```python
from build123d import *

# Parameters (mm, degrees)
F1_DEPTH = 40.64
F3_DEPTH = 38.608
F5_DEPTH = 4.7752
F6_R     = 1.35255
F7_DEPTH = 4.7752


# Not quite as in the source:
# - a feature names something its author has since deleted; it is built from what else it names


with BuildPart() as f1:
    # F0 (on Top) → F1 (new body)
    with BuildSketch(Plane.XY):
        with BuildLine():
            ThreePointArc((0, 2), (0.5857864376, 0.5857864376), (2, 0))
            Line((2, 0), (50.07, 0))
            ThreePointArc((50.07, 0), (51.4842135624, 0.5857864376), (52.07, 2))
            Line((52.07, 2), (52.07, 36.1))
            ThreePointArc((52.07, 36.1), (51.4842135624, 37.5142135624), (50.07, 38.1))
            Line((50.07, 38.1), (2, 38.1))
            ThreePointArc((2, 38.1), (0.5857864376, 37.5142135624), (0, 36.1))
            Line((0, 36.1), (0, 2))
        make_face()
    extrude(amount=F1_DEPTH)

    # F2 (on face) → F3 (cut)
    with BuildSketch(Plane.XY.offset(40.64)):
        with BuildLine():
            Line((49.27, 36.3), (2.8, 36.3))
            ThreePointArc((2.8, 36.3), (2.0928932188, 36.0071067812), (1.8, 35.3))
            Line((1.8, 35.3), (1.8, 2.8))
            ThreePointArc((1.8, 2.8), (2.0928932188, 2.0928932188), (2.8, 1.8))
            Line((2.8, 1.8), (49.27, 1.8))
            ThreePointArc((49.27, 1.8), (49.9771067812, 2.0928932188), (50.27, 2.8))
            Line((50.27, 2.8), (50.27, 35.3))
            ThreePointArc((50.27, 35.3), (49.9771067812, 36.0071067812), (49.27, 36.3))
        make_face()
    extrude(amount=-F3_DEPTH, mode=Mode.SUBTRACT)

    # F4 (on face) → F5 (join)
    with BuildSketch(Plane(origin=(0, 0, 0), x_dir=(1, 0, 0), z_dir=(0, 0, -1))):
        with BuildLine():
            ThreePointArc((52.07, -2), (51.4842135624, -0.5857864376), (50.07, 0))
            Line((50.07, 0), (46.26, 0))
            Line((46.26, 0), (46.26, -2))
            ThreePointArc((46.26, -2), (47.3759231637, -4.6940768363), (50.07, -5.81))
            Line((50.07, -5.81), (52.07, -5.81))
            Line((52.07, -5.81), (52.07, -2))
        make_face()
        with BuildLine():
            Line((46.26, -36.1), (46.26, -38.1))
            Line((46.26, -38.1), (50.07, -38.1))
            ThreePointArc((50.07, -38.1), (51.4842135624, -37.5142135624), (52.07, -36.1))
            Line((52.07, -36.1), (52.07, -32.29))
            Line((52.07, -32.29), (50.07, -32.29))
            ThreePointArc((50.07, -32.29), (47.3759231637, -33.4059231637), (46.26, -36.1))
        make_face()
        with BuildLine():
            ThreePointArc((5.81, -36.1), (4.6940768363, -33.4059231637), (2, -32.29))
            Line((2, -32.29), (0, -32.29))
            Line((0, -32.29), (0, -36.1))
            ThreePointArc((0, -36.1), (0.5857864376, -37.5142135624), (2, -38.1))
            Line((2, -38.1), (5.81, -38.1))
            Line((5.81, -38.1), (5.81, -36.1))
        make_face()
        with BuildLine():
            Line((5.81, 0), (2, 0))
            ThreePointArc((2, 0), (0.5857864376, -0.5857864376), (0, -2))
            Line((0, -2), (0, -5.81))
            Line((0, -5.81), (2, -5.81))
            ThreePointArc((2, -5.81), (4.6940768363, -4.6940768363), (5.81, -2))
            Line((5.81, -2), (5.81, 0))
        make_face()
    extrude(amount=-F5_DEPTH)

    # F6 (on face) → F7 (cut, through all)
    with BuildSketch(Plane(origin=(0, 0, 0), x_dir=(1, 0, 0), z_dir=(0, 0, -1))):
        with Locations((48.7198709242, -3.3501290758)):
            Circle(F6_R)
        with Locations((3.3501290758, -3.3501290758)):
            Circle(F6_R)
        with Locations((3.3501290758, -34.7498709242)):
            Circle(F6_R)
        with Locations((48.7198709242, -34.7498709242)):
            Circle(F6_R)
    extrude(amount=-F7_DEPTH, mode=Mode.SUBTRACT)


solid = f1.part
```
Design review of the part built by this model. Coordinates are the model's own, in mm. A direction names the side the tool comes from. Coordinates: 2 decimals unless noted, no trailing zeros. Order: outer loops, then holes, each group sorted by start corner. A loop starts at its lowest first (then second) coordinate and runs counter-clockwise, first axis right, second up.
1) Wall thickness on line 1 along X through (y, z) = (20.5, 27.5); line 2 along Y through (x, z) = (43, 29); line 3 along Z through (x, y) = (45.5, 7): over which ranges is each line inside the solid? List them lowest first.
2) Clearance check with flat-ended pins moving along their axes: pin 1 (3 mm diameter, centred on x = 47.5, y = 34, fed in from +Z); pin 2 (10 mm diameter, centred on x = 11.5, y = 12.5, fed in from +Z). State where each tip first meets the part, or that it passes through.
3) Take a section at C-C, the plane x = 19. Give the boundary of the cut face in (y, z).
4) Take a section at D-D, the plane z = 3.5. Give the boundary of the cut face in (x, y).
5) Take a section at B-B, the plane y = 11.5. Give the boundary of the cut face in (x, z), and give its area (3 significant figures).
6) Mouldability with a two-part tool opening along X and no side actions: class faces 1 (the cylindrical face through (4.64, 2.94, 2.35)), 2 (the flat face through (52.07, 19, 20)), 3 (the flat face through (26, 0, 20)) as +X half, -X half, draft (parallel to the pull), parting line (faces both ways), or undercut.
7) Take a section at A-A, the plane z = 24.5. Give the boundary of the cut face in (x, y), and give its area (3 significant figures).
8) For faces 4 (the cylindrical face through (51.5, 0.6, 20)), 5 (the flat face through (47, 35, 4.775)), list the 3-axis set-ups (+Z, -Z, +X, -X, +Y, -Y) from which the entire face can be reached by the end or side of a thin tool; tool diameter is ignored.
Returned:
1. line 1: x = 0 to 1.8, 50.27 to 52.07
1. line 2: y = 0 to 1.8, 36.3 to 38.1
1. line 3: z = 0 to 2.03
2. pin 1: stops at z = 4.78
2. pin 2: stops at z = 2.03
3. outline: (0, 0) - (38.1, 0) - (38.1, 40.64) - (36.3, 40.64) - (36.3, 2.03) - (1.8, 2.03) - (1.8, 40.64) - (0, 40.64) - close
4. outline: (0, 2) arc R2 ccw to (2, 0) - (50.07, 0) arc R2 ccw to (52.07, 2) - (52.07, 36.1) arc R2 ccw to (50.07, 38.1) - (2, 38.1) arc R2 ccw to (0, 36.1) - close; hole (1.8, 5.81) - (2, 5.81) arc R3.81 cw to (5.81, 2) - (5.81, 1.8) - (46.26, 1.8) - (46.26, 2) arc R3.81 cw to (50.07, 5.81) - (50.27, 5.81) - (50.27, 32.29) - (50.07, 32.29) arc R3.81 cw to (46.26, 36.1) - (46.26, 36.3) - (5.81, 36.3) - (5.81, 36.1) arc R3.81 cw to (2, 32.29) - (1.8, 32.29) - close; hole circle Ø2.71 at (3.35, 3.35); hole circle Ø2.71 at (3.35, 34.75); hole circle Ø2.71 at (48.72, 3.35); hole circle Ø2.71 at (48.72, 34.75)
5. outline: (0, 0) - (52.07, 0) - (52.07, 40.64) - (50.27, 40.64) - (50.27, 2.03) - (1.8, 2.03) - (1.8, 40.64) - (0, 40.64) - close
5. area: 245 mm2
6. face 1: undercut
6. face 2: +X half
6. face 3: draft
7. outline: (0, 2) arc R2 ccw to (2, 0) - (50.07, 0) arc R2 ccw to (52.07, 2) - (52.07, 36.1) arc R2 ccw to (50.07, 38.1) - (2, 38.1) arc R2 ccw to (0, 36.1) - close; hole (1.8, 2.8) arc R1 ccw to (2.8, 1.8) - (49.27, 1.8) arc R1 ccw to (50.27, 2.8) - (50.27, 35.3) arc R1 ccw to (49.27, 36.3) - (2.8, 36.3) arc R1 ccw to (1.8, 35.3) - close
7. area: 309 mm2
8. face 4: +Z, -Z, +X, -Y
8. face 5: +Z
